Check sheet for the drawn part. Datum: minimum x, y, z corner. Units: mm. A direction names the side the tool comes from. Coordinates: 2 decimals unless noted, no trailing zeros. Loops run counter-clockwise (first coordinate to the right, second up) from the corner with the lowest first, then second, coordinate; pieces in that order, holes last. Notation, with made-up numbers: M 26,68 L 64,68 A13 ccw 64,93 Z; hole C 80,38.5 d5. An arc over 180 degrees is marked long. Answer as CSV lines item,"result". Start each with the question number.
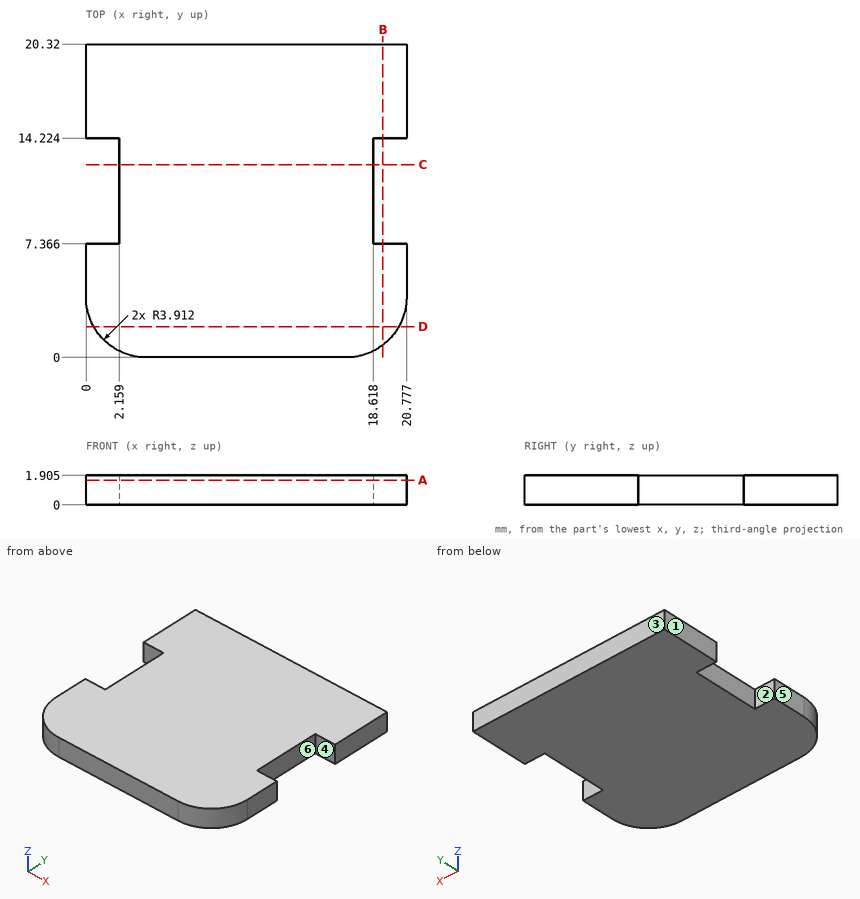
Item 1: Material ranges on line 1 (X direction, y = 11.5, z = 1.6); line 2 (Y direction, x = 17, z = 0.35); line 3 (Y direction, x = 2, z = 0.3) (1 decimal), recorded low to high. Write a range as from..to.
Item 2: Sectioned sample at A-A, the plane z = 1.6. Record the boundary of the cut face in (x, y) (1 decimal), and give its area (3 significant figures).
Item 3: Go/stop test with a flat-tipped pin: pin 1 (1 mm diameter, centred on y = 9.5, z = 1, fed in from -X). Record where the tip stops, or that it passes through.
Item 4: Release check for a two-part mould opening along Y. For the marked faces 3, 4, 5 and 6 record: released by +Y, released by -Y, zero draft, split by the parting line, or undercut.
Item 5: Set-up check for the marked faces 1 and 2: record each of +Z, -Z, +X, -X, +Y, -Y from which the full face is reachable in a straight line by a thin tool's end or side.
Item 6: Sectioned sample at B-B, the plane x = 19.25. Record the boundary of the cut face in (y, z) (1 decimal).
Item 7: Sectioned sample at D-D, the plane y = 2. Record the boundary of the cut face in (x, z) (1 decimal).
Item 8: Sectioned sample at C-C, the plane y = 12.5. Record the boundary of the cut face in (x, z) (1 decimal).
Reply:
1,line 1,"2.16..18.62"
1,line 2,"0..20.32"
1,line 3,"0.5..7.4, 14.2..20.3"
2,outline,"M 0,3.9 A3.9 ccw 3.9,0 L 16.9,0 A3.9 ccw 20.8,3.9 L 20.8,7.4 L 18.6,7.4 L 18.6,14.2 L 20.8,14.2 L 20.8,20.3 L 0,20.3 L 0,14.2 L 2.2,14.2 L 2.2,7.4 L 0,7.4 Z"
2,area,"386 mm²"
3,pin 1,"x = 2.16"
4,face 3,"released by +Y"
4,face 4,"undercut"
4,face 5,"zero draft"
4,face 6,"undercut"
5,face 1,"+Z, -Z, -X, +Y, -Y"
5,face 2,"+Z, -Z, -X"
6,outline,"M 0.8,0 L 7.4,0 L 7.4,1.9 L 0.8,1.9 Z; M 14.2,0 L 20.3,0 L 20.3,1.9 L 14.2,1.9 Z"
7,outline,"M 0.5,0 L 20.3,0 L 20.3,1.9 L 0.5,1.9 Z"
8,outline,"M 2.2,0 L 18.6,0 L 18.6,1.9 L 2.2,1.9 Z"
